For this review, take the finished solid that the model builds, in its own axes (mm). Round coordinates to 2 decimals unless told otherwise and drop trailing zeros. Loops run counter-clockwise (first coordinate to the right, second up) from the corner with the lowest first, then second, coordinate; pieces in that order, holes last. Notation, with made-up numbers: M 26,36 L 47,36 A24 ccw 47,63 Z; hole C 59.5,-33 d11. An arc over 180 degrees is marked long. One line per question, with ' | ' between items. Start each with the question number.
1) For probe 1 along Y at (x, z) = (25, 0.6); probe 2 along X at (y, z) = (-77, 0.6); probe 3 along X at (y, z) = (-26, 0.3), list the stretches that pass through material, from the lowest coordinate up. Write a range as from..to.
2) Mouldability with a two-part tool opening along X and no side actions: class faces 1 (the face through (76, -99, 2)), 2 (the face through (25.59, -70.54, 0.99)), 3 (the face through (124, -126, 1)) as pulls with the +X half, pulls with the -X half, needs draft (parallel to the pull), parting line crosses it, or undercut.
3) We need section B-B (y = -175). Give the boundary of the cut face in (x, z), and give its area (3 significant figures).
4) We need section C-C (y = -125). Give the boundary of the cut face in (x, z), and give its area (3 significant figures).
5) We need section D-D (x = 75). Give the boundary of the cut face in (y, z).
6) We need section A-A (x = 175). Give the boundary of the cut face in (y, z).
```python
from build123d import *

# Parameters (mm, degrees)
EXTRUDE_1_DEPTH   = 2
CHAMFER_1_SIZE    = 2
HOLE_WIZARD_M81_D = 9


with BuildPart() as part:
    # Эскиз1 → Бобышка-Вытянуть1 (new body)
    with BuildSketch(Plane.XY):
        Polygon((0, 0), (0, -200), (50, -200), (200, -50), (200, 0), align=None)
    extrude(amount=EXTRUDE_1_DEPTH)

    # Фаска1
    chamfer_1_edges = [part.edges().sort_by_distance(p)[0] for p in [
        (200, 0, 1),
        (0, -200, 1),
        (0, 0, 1),
    ]]
    chamfer(chamfer_1_edges, length=CHAMFER_1_SIZE)

    # Отверстие с зазором M81 (through all)
    with Locations(Plane.XY.offset(2)):
        with Locations((25, -25), (75, -25), (125, -25), (175, -25), (25, -75), (25, -125), (25, -175), (75, -125), (125, -75), (75, -75)):
            Hole(HOLE_WIZARD_M81_D / 2)


solid = part.part
```
Answers below:
1) probe 1: -200..-179.5, -170.5..-129.5, -120.5..-79.5, -70.5..-29.5, -20.5..0 | probe 2: 0..20.97, 29.03..70.97, 79.03..120.97, 129.03..173 | probe 3: 0..20.61, 29.39..70.61, 79.39..120.61, 129.39..170.61, 179.39..200
2) face 1: needs draft | face 2: undercut | face 3: pulls with the +X half
3) outline: M 0,0 L 20.5,0 L 20.5,2 L 0,2 Z; M 29.5,0 L 75,0 L 75,2 L 29.5,2 Z | area: 132 mm^2
4) outline: M 0,0 L 20.5,0 L 20.5,2 L 0,2 Z; M 29.5,0 L 70.5,0 L 70.5,2 L 29.5,2 Z; M 79.5,0 L 125,0 L 125,2 L 79.5,2 Z | area: 214 mm^2
5) outline: M -175,0 L -129.5,0 L -129.5,2 L -175,2 Z; M -120.5,0 L -79.5,0 L -79.5,2 L -120.5,2 Z; M -70.5,0 L -29.5,0 L -29.5,2 L -70.5,2 Z; M -20.5,0 L 0,0 L 0,2 L -20.5,2 Z
6) outline: M -75,0 L -29.5,0 L -29.5,2 L -75,2 Z; M -20.5,0 L 0,0 L 0,2 L -20.5,2 Z
